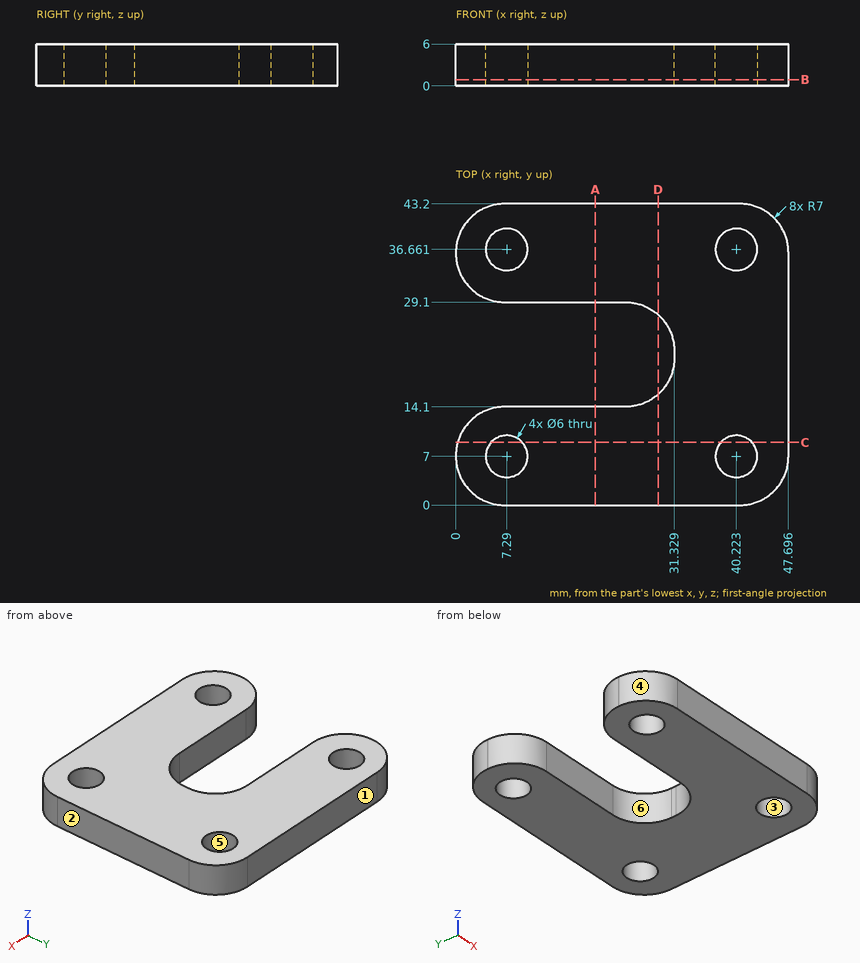
Drawing for the job (mm, zero at the part's lowest x, y, z). A direction names the side the tool comes from. Give positions to 0.01 mm unless a question says otherwise; leave off trailing zeros. Loops run counter-clockwise (first coordinate to the right, second up) from the corner with the lowest first, then second, coordinate; pieces in that order, holes last.
Item 1: Drop a flat-ended pin along its axis: P1, Ø5, axis at x = 40.22, y = 7, coming from the -Z side. Give the stop position or say it passes through.
Check values:
P1: passes through
Item 2: Slice it at B-B (z = 0.9). Write the cut outline in (x, y), plus the area to 3 significant figures.
Check values:
outline: (0, 7) arc R7 ccw to (7, 0) - (40.7, 0) arc R7 ccw to (47.7, 7) - (47.7, 36.2) arc R7 ccw to (40.7, 43.2) - (7, 43.2) arc R7 ccw to (0, 36.2) - (0, 36.1) arc R7 ccw to (7, 29.1) - (24.33, 29.1) arc R7 cw to (31.33, 22.1) - (31.33, 21.1) arc R7 cw to (24.33, 14.1) - (7, 14.1) arc R7 ccw to (0, 7.1) - close; hole circle Ø6 at (7.29, 7); hole circle Ø6 at (7.29, 36.66); hole circle Ø6 at (40.22, 7); hole circle Ø6 at (40.22, 36.66)
area: 1,440 mm2
Item 3: Which spindle directions (+Z, -Z, +X, -X, +Y, -Y) get a long thin tool onto all of the face, cutting with end or side? Do the marked faces 5 and 6. Say none if no direction does.
Check values:
face 5: +Z, -Z
face 6: +Z, -Z, -X
Item 4: Slice it at D-D (x = 29). Write the cut outline in (y, z).
Check values:
outline: (0, 0) - (15.89, 0) - (15.89, 6) - (0, 6) - close; (27.31, 0) - (43.2, 0) - (43.2, 6) - (27.31, 6) - close
Item 5: Mould opens along X. For the marked faces 1, 2, 3 and 4 say: +X half, -X half, draft (parallel to the pull), parting line (faces both ways), or undercut.
Check values:
face 1: draft
face 2: +X half
face 3: undercut
face 4: -X half
Item 6: Slice it at C-C (y = 9). Write the cut outline in (x, z).
Check values:
outline: (0.26, 0) - (5.05, 0) - (5.05, 6) - (0.26, 6) - close; (9.53, 0) - (37.99, 0) - (37.99, 6) - (9.53, 6) - close; (42.46, 0) - (47.7, 0) - (47.7, 6) - (42.46, 6) - close
Item 7: Slice it at A-A (x = 20). Write the cut outline in (y, z), plus the area to 3 significant figures.
Check values:
outline: (0, 0) - (14.1, 0) - (14.1, 6) - (0, 6) - close; (29.1, 0) - (43.2, 0) - (43.2, 6) - (29.1, 6) - close
area: 169 mm2
Item 8: Drill centre lines: line 1 along Y through (x, z) = (40.5, 2.1) (1 decimal); line 2 along Y through (x, z) = (11.5, 3.25); line 3 along X through (y, z) = (5.5, 1.8) (1 decimal). Where is each one in solid material? Low to high.
Check values:
line 1: y = 0 to 4, 10 to 33.7, 39.6 to 43.2
line 2: y = 0 to 14.1, 29.1 to 43.2
line 3: x = 0.2 to 4.7, 9.9 to 37.6, 42.8 to 47.5
